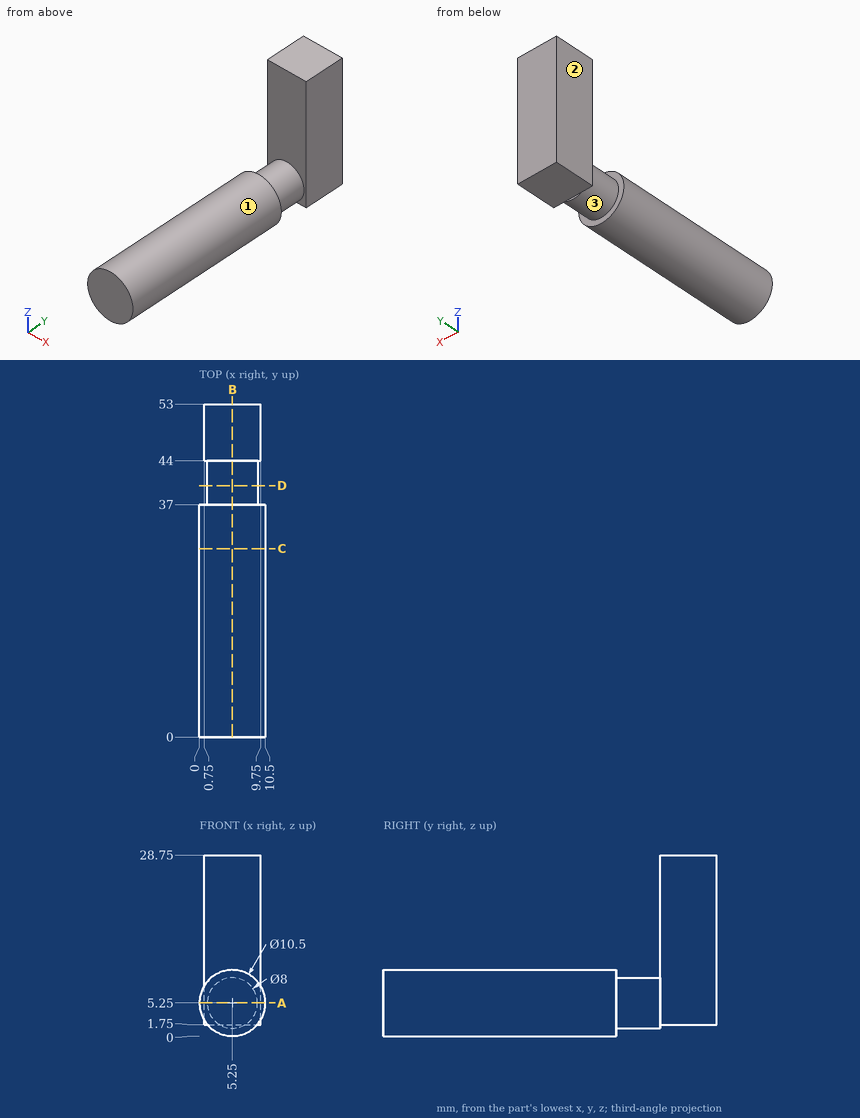
Could you check a few things on this drawing? It's one solid part, dimensions in mm from its lowest x, y, z. A direction names the side the tool comes from. Coordinates: 2 decimals unless noted, no trailing zeros. Write each loop counter-clockwise with the first axis right and the second up, starting at its lowest first coordinate (ties: lowest second). Pieces come first, ordered by that corner, then holes.
1) If we section it at D-D (y = 40): List the corners of the cut face in (x, z) for me, plus the area to 3 significant figures.
Filled in:
outline: circle Ø8 at (5.25, 5.25)
area: 50.3 mm2
2) If I drill on line 1 (Y direction, x = 4, z = 21.25); line 2 (X direction, y = 45, z = 15); line 3 (Z direction, x = 6, y = 45), over which ranges is the centre line in solid material (lowest first)?
Filled in:
line 1: y = 44 to 53
line 2: x = 0.75 to 9.75
line 3: z = 1.75 to 28.75
3) I'm going to push flat-ended pins straight in: pin 1 (6 mm diameter, centred on y = 24.5, z = 16, fed in from +X) (1 decimal); pin 2 (7 mm diameter, centred on y = 46.5, z = 11, fed in from +X); pin 3 (4.5 mm diameter, centred on y = 49.5, z = 18, fed in from -X); pin 4 (4.5 mm diameter, centred on x = 6, y = 50.5, fed in from -Z). Where does each tip first touch, or does it pass through?
Filled in:
pin 1: passes through
pin 2: stops at x = 9.75
pin 3: stops at x = 0.75
pin 4: stops at z = 1.75
4) If we section it at C-C (y = 30): List the corners of the cut face in (x, z) for me, plus the area to 3 significant figures.
Filled in:
outline: circle Ø10.5 at (5.25, 5.25)
area: 86.6 mm2
5) If we section it at A-A (z = 5.25): List the corners of the cut face in (x, y) for me, plus the area to 4 significant figures.
Filled in:
outline: (0, 0) - (10.5, 0) - (10.5, 37) - (9.25, 37) - (9.25, 44) - (9.75, 44) - (9.75, 53) - (0.75, 53) - (0.75, 44) - (1.25, 44) - (1.25, 37) - (0, 37) - close
area: 525.5 mm2
6) Which directions (+Z, -Z, +X, -X, +Y, -Y) give clear straight access to the entire face, cutting with the end or side of a thin tool? Please do the marked faces 1, 2 and 3.
Filled in:
face 1: -Y
face 2: +Z, -Z, -X, +Y
face 3: none
7) If we section it at B-B (x = 5.25): List the corners of the cut face in (y, z) for me.
Filled in:
outline: (0, 0) - (37, 0) - (37, 1.25) - (44, 1.25) - (44, 1.75) - (53, 1.75) - (53, 28.75) - (44, 28.75) - (44, 9.25) - (37, 9.25) - (37, 10.5) - (0, 10.5) - close
